Part print with two shaded views. Sizes in mm from the minimum x, y, z corner. A direction names the side the tool comes from. Coordinates: 2 decimals unless noted, no trailing zeros. Write each loop counter-clockwise with the first axis right and the second up, starting at its lowest first coordinate (ties: lowest second). Pieces come first, ordered by that corner, then holes. Notation, with made-up numbers: M 32.5,65.5 L 44.5,65.5 A25 cw 44.5,80.5 Z; hole C -16,7 d9. An arc over 180 degrees is marked long. Answer in a Markdown table with one row per item. Add a question column.
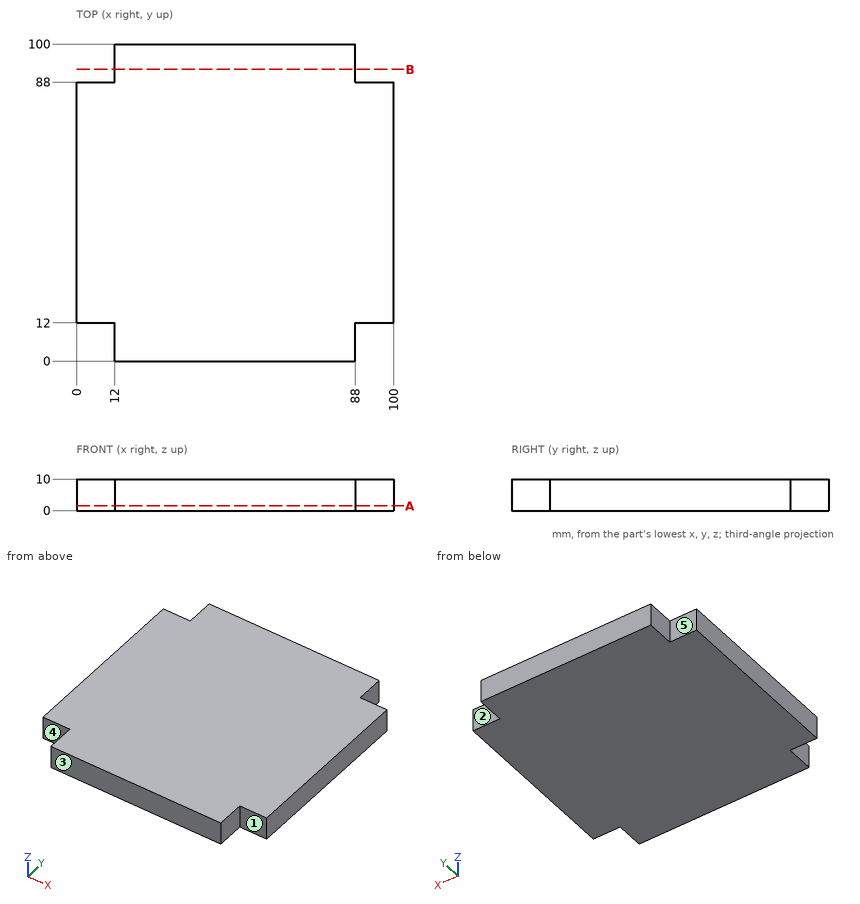
1) Slice it at A-A (z = 1.5). Give the cut face in (x, y), then the cut area to 3 significant figures.
2) Flat gauge pins, fed straight in: pin 1 Ø5 at (x, z) = (4.5, 3) entering from +Y; pin 2 Ø5 at (y, z) = (92.5, 5) entering from -X; pin 3 Ø5 at (y, z) = (93, 7.5) entering from +X. Where does each tip first touch, or does it go through?
3) Which spindle directions (+Z, -Z, +X, -X, +Y, -Y) get a long thin tool onto all of the face, cutting with end or side? Do the marked faces 1, 2, 3, 4 and 5. Say none if no direction does.
4) Drill centre line: probe 1 along X at (y, z) = (95, 2.25). Where is it in solid material? Low to high.
5) Slice it at B-B (y = 92). Give the cut face in (x, z), then the cut area to 3 significant figures.
Ans:
| question | item | result |
|---|---|---|
| 1 | outline | M 0,12 L 12,12 L 12,0 L 88,0 L 88,12 L 100,12 L 100,88 L 88,88 L 88,100 L 12,100 L 12,88 L 0,88 Z |
| 1 | area | 9,420 mm2 |
| 2 | pin 1 | stops at y = 88 |
| 2 | pin 2 | stops at x = 12 |
| 2 | pin 3 | stops at x = 88 |
| 3 | face 1 | +Z, -Z, +X, -Y |
| 3 | face 2 | +Z, -Z, +X, +Y |
| 3 | face 3 | +Z, -Z, +X, -X, -Y |
| 3 | face 4 | +Z, -Z, -X, -Y |
| 3 | face 5 | +Z, -Z, -X, +Y |
| 4 | probe 1 | x = 12 to 88 |
| 5 | outline | M 12,0 L 88,0 L 88,10 L 12,10 Z |
| 5 | area | 760 mm2 |
